Part model, mm, in its own coordinate system. Face numbers are marked on the shaded views. A direction names the side the tool comes from. Round coordinates to 2 decimals unless told otherwise and drop trailing zeros. Order: outer loops, then holes, each group sorted by start corner. A loop starts at its lowest first (then second) coordinate and runs counter-clockwise, first axis right, second up. Notation, with made-up numbers: (48, 88.5) -> (80, 88.5) arc R16 cw to (80, 110.5) -> close; hole circle Ø11 at (-36, 35). An arc over 180 degrees is marked (long way). Return JSON: item names as keys, results as strings. Group by question number.
from build123d import *

# Parameters (mm, degrees)
BOSS_EXTRUDE1_DEPTH  = 30.81
BOSS_EXTRUDE2_DEPTH  = 0.5
BOSS_EXTRUDE3_DEPTH  = 5.4
CUT_EXTRUDE1_REACH   = 22.746
BOSS_EXTRUDE14_REACH = 24.041
SKETCH15_R           = 2.25
HOLE1_D              = 2.156
CHAMFER1_SIZE        = 0.25
SKETCH19_R           = 0.335
BOSS_EXTRUDE15_DEPTH = 4.99618


with BuildPart() as part:
    # Sketch1 → Boss-Extrude1 (new body)
    with BuildSketch(Plane(origin=(-15.405, 0, 0), x_dir=(0, -1, 0), z_dir=(-1, 0, 0))):
        Polygon((-12.58, -3.6), (0, -3.6), (0, 0), (-3.599999999, 0), (-12.58, 0), align=None)
    extrude(amount=-BOSS_EXTRUDE1_DEPTH)

    # Sketch2 → Boss-Extrude2 (add)
    with BuildSketch(Plane(origin=(0, 0, -4.1), x_dir=(-1, 0, 0), z_dir=(0, 0, -1))):
        with BuildLine():
            Line((-15.155, 11.83), (-15.155, 0.75))
            ThreePointArc((-15.155, 0.75), (-15.008553391, 0.396446609), (-14.655, 0.25))
            Line((-14.655, 0.25), (14.655, 0.25))
            ThreePointArc((14.655, 0.25), (15.008553391, 0.396446609), (15.155, 0.75))
            Line((15.155, 0.75), (15.155, 11.83))
            ThreePointArc((15.155, 11.83), (15.008553391, 12.183553391), (14.655, 12.33))
            Line((14.655, 12.33), (-14.655, 12.33))
            ThreePointArc((-14.655, 12.33), (-15.008553391, 12.183553391), (-15.155, 11.83))
        make_face()
    extrude(amount=-BOSS_EXTRUDE2_DEPTH)

    # Sketch3 → Boss-Extrude3 (add)
    with BuildSketch(Plane(origin=(0, 0, -9.5), x_dir=(-1, 0, 0), z_dir=(0, 0, -1))):
        with BuildLine():
            Line((-8.887403877, 9.154527733), (-7.785360247, 2.904527733))
            ThreePointArc((-7.785360247, 2.904527733), (-7.272330032, 2.015933335), (-6.308148618, 1.665))
            Line((-6.308148618, 1.665), (6.308148618, 1.665))
            ThreePointArc((6.308148618, 1.665), (7.272330032, 2.015933335), (7.785360247, 2.904527733))
            Line((7.785360247, 2.904527733), (8.887403877, 9.154527733))
            ThreePointArc((8.887403877, 9.154527733), (8.559258912, 10.379181415), (7.410192247, 10.915))
            Line((7.410192247, 10.915), (-7.410192247, 10.915))
            ThreePointArc((-7.410192247, 10.915), (-8.559258912, 10.379181415), (-8.887403877, 9.154527733))
        make_face()
    extrude(amount=-BOSS_EXTRUDE3_DEPTH)

    # Sketch4 → Cut-Extrude1 (cut, up to next)
    with BuildSketch(Plane.XY.offset(-3.6), mode=Mode.PRIVATE) as cut_extrude1_sk1:
        with BuildLine():
            Line((7.410192247, 10.415), (-7.410192247, 10.415))
            ThreePointArc((-7.410192247, 10.415), (-8.17623669, 10.05778761), (-8.395, 9.241351822))
            Line((-8.395, 9.241351822), (-7.292956371, 2.991351822))
            ThreePointArc((-7.292956371, 2.991351822), (-6.950936227, 2.398955557), (-6.308148618, 2.165))
            Line((-6.308148618, 2.165), (6.308148618, 2.165))
            ThreePointArc((6.308148618, 2.165), (6.950936227, 2.398955557), (7.292956371, 2.991351822))
            Line((7.292956371, 2.991351822), (8.395, 9.241351822))
            ThreePointArc((8.395, 9.241351822), (8.17623669, 10.05778761), (7.410192247, 10.415))
        make_face()
    cut_extrude1_tool1 = extrude(cut_extrude1_sk1.sketch, amount=-CUT_EXTRUDE1_REACH, mode=Mode.PRIVATE) & part.part
    add(cut_extrude1_tool1.solids().sort_by_distance((0, 6.407458, -3.6))[0], mode=Mode.SUBTRACT)

    # Sketch15 → Boss-Extrude14 (add, up to next)
    with BuildSketch(Plane(origin=(0, 0, -9.5), x_dir=(-1, 0, 0), z_dir=(0, 0, -1)), mode=Mode.PRIVATE) as boss_extrude14_sk1:
        with Locations((-12.495, 6.29)):
            Circle(SKETCH15_R)
    boss_extrude14_tool1 = extrude(boss_extrude14_sk1.sketch, amount=-BOSS_EXTRUDE14_REACH, mode=Mode.PRIVATE) - part.part
    # Sketch15 → Boss-Extrude14 (add, up to next)
    with BuildSketch(Plane(origin=(0, 0, -9.5), x_dir=(-1, 0, 0), z_dir=(0, 0, -1)), mode=Mode.PRIVATE) as boss_extrude14_sk2:
        with Locations((12.495, 6.29)):
            Circle(SKETCH15_R)
    boss_extrude14_tool2 = extrude(boss_extrude14_sk2.sketch, amount=-BOSS_EXTRUDE14_REACH, mode=Mode.PRIVATE) - part.part
    add(boss_extrude14_tool1.solids().sort_by_distance((12.495, 6.29, -9.5))[0])
    add(boss_extrude14_tool2.solids().sort_by_distance((-12.495, 6.29, -9.5))[0])

    # Hole1 (through all)
    with Locations(Plane(origin=(0, 0, -9.5), x_dir=(-1, 0, 0), z_dir=(0, 0, -1))):
        with Locations((12.495, 6.29), (-12.495, 6.29)):
            Hole(HOLE1_D / 2)

    # Chamfer1
    chamfer1_edges = [part.edges().sort_by_distance(p)[0] for p in [
        (14.745, 6.29, -9.5),
        (-10.245, 6.29, -9.5),
        (11.417, 6.29, -9.5),
        (-13.573, 6.29, -9.5),
    ]]
    chamfer(chamfer1_edges, length=CHAMFER1_SIZE)

    # Sketch19 → Boss-Extrude15 (add)
    with BuildSketch(Plane(origin=(0, 0, -3.6), x_dir=(-1, 0, 0), z_dir=(0, 0, -1))):
        with Locations(Location((-5.48, 7.71, 0), (0, 0, 180))):
            Circle(SKETCH19_R)
        with Locations(Location((-2.74, 7.71, 0), (0, 0, 180))):
            Circle(SKETCH19_R)
        with Locations(Location((0, 7.71, 0), (0, 0, 180))):
            Circle(SKETCH19_R)
        with Locations(Location((2.74, 7.71, 0), (0, 0, 180))):
            Circle(SKETCH19_R)
        with Locations(Location((5.48, 7.71, 0), (0, 0, 180))):
            Circle(SKETCH19_R)
        with Locations(Location((4.11, 4.87, 0), (0, 0, 180))):
            Circle(SKETCH19_R)
        with Locations(Location((1.37, 4.87, 0), (0, 0, 180))):
            Circle(SKETCH19_R)
        with Locations(Location((-1.37, 4.87, 0), (0, 0, 180))):
            Circle(SKETCH19_R)
        with Locations(Location((-4.11, 4.87, 0), (0, 0, 180))):
            Circle(SKETCH19_R)
    extrude(amount=BOSS_EXTRUDE15_DEPTH)


solid = part.part
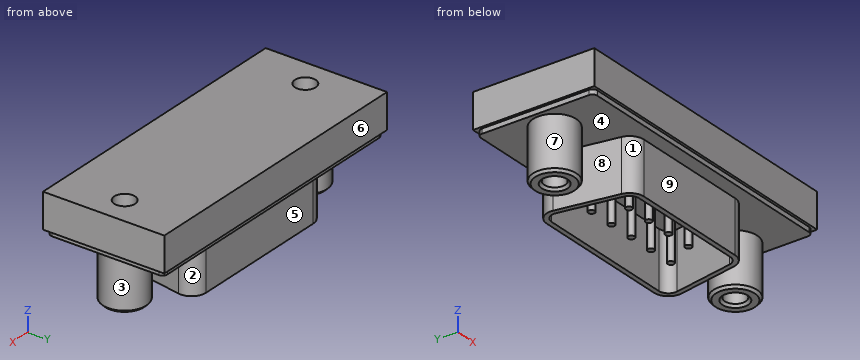
(1) Saw through at A-A, the plane z = -4.5. State how many separate pieces and enclosed holes the cut face has, and give its area (3 significant figures).
(2) Tool access for the marked faces 5, 6, 7, 8 and 9: list every direction of +Z, -Z, +X, -X, +Y, -Y with a clear straight run to the whole face (end or side of a thin tool).
(3) Saw through at B-B, the plane x = 5.48. List the corners of the cut face in (y, z) (3 decimals).
(4) Pin check, flat tips, straight feed: P1, Ø3, axis at x = -3.5, y = 8.5, coming from the -Z side; P2, Ø3, axis at x = 0, z = -5.5, coming from the +Y side; P3, Ø4, axis at x = -3.5, y = 3.5, coming from the -Z side; P4, Ø2, axis at y = 6, z = -7, coming from the +X side (3 decimals). Stop position of each tip, or through.
(5) Probe L1, parallel to X at y = 6.25, z = -2.25 (3 decimals); L2, parallel to Y at x = 4, z = -6.75 (3 decimals); L3, parallel to Y at x = -6, z = -8 (3 decimals). List the from-to ranges inside material, lowest first. Write a range as [from, to].
(6) Saw through at C-C, the plane z = -1.5. List the corners of the cut face in (x, y) (3 decimals), and give its area (3 significant figures).
(7) Mould opens along X. For the marked faces 1, 2, 3 and 4 say: pulls with the +X half, pulls with the -X half, needs draft (parallel to the pull), parting line crosses it, or undercut.
Results are:
{
 "1": {"separate pieces": "12", "enclosed holes": "3", "area": "51.7 mm^2"},
 "2": {"face 5": "-Z, +X, -X, +Y", "face 6": "+Z, -Z, +X, -X, +Y", "face 7": "-Z", "face 8": "-Z, -Y", "face 9": "-Z, +X, -X, -Y"},
 "3": {"outline": "(0, -3.6) -> (0.25, -3.6) -> (0.25, -4.1) -> (1.665, -4.1) -> (1.665, -9.5) -> (2.165, -9.5) -> (2.165, -3.6) -> (7.375, -3.6) -> (7.375, -8.596) -> (8.045, -8.596) -> (8.045, -3.6) -> (10.415, -3.6) -> (10.415, -9.5) -> (10.915, -9.5) -> (10.915, -4.1) -> (12.33, -4.1) -> (12.33, -3.6) -> (12.58, -3.6) -> (12.58, 0) -> (0, 0) -> close"},
 "4": {"P1": "stops at z = -8.6", "P2": "stops at y = 12.33", "P3": "stops at z = -9.5", "P4": "stops at x = 14.745"},
 "5": {"L1": "x = [-15.405, -13.572], [-11.418, 11.418], [13.572, 15.405]", "L2": "y = [1.665, 2.165], [4.554, 5.186], [10.415, 10.915]", "L3": "y = [1.665, 2.165], [10.415, 10.915]"},
 "6": {"outline": "(-15.405, 0) -> (15.405, 0) -> (15.405, 12.58) -> (-15.405, 12.58) -> close; hole circle Ø2.156 at (-12.495, 6.29); hole circle Ø2.156 at (12.495, 6.29)", "area": "380 mm^2"},
 "7": {"face 1": "pulls with the -X half", "face 2": "pulls with the +X half", "face 3": "undercut", "face 4": "undercut"}
}
